Design review of the part shown in the three views and the two pictorial views. Dimensions are in mm from the part's minimum x, y and z. Give positions to 0.01 mm unless a question says otherwise; leave off trailing zeros. Write each loop counter-clockwise with the first axis right and the second up, starting at its lowest first coordinate (ties: lowest second). Pieces come first, ordered by that corner, then holes. Notation, with made-up numbers: M 43,21 L 67,21 A26 ccw 67,44 Z; hole C -11.75,-34.75 d4. An arc over 180 degrees is marked long. Write item = value, one per line.
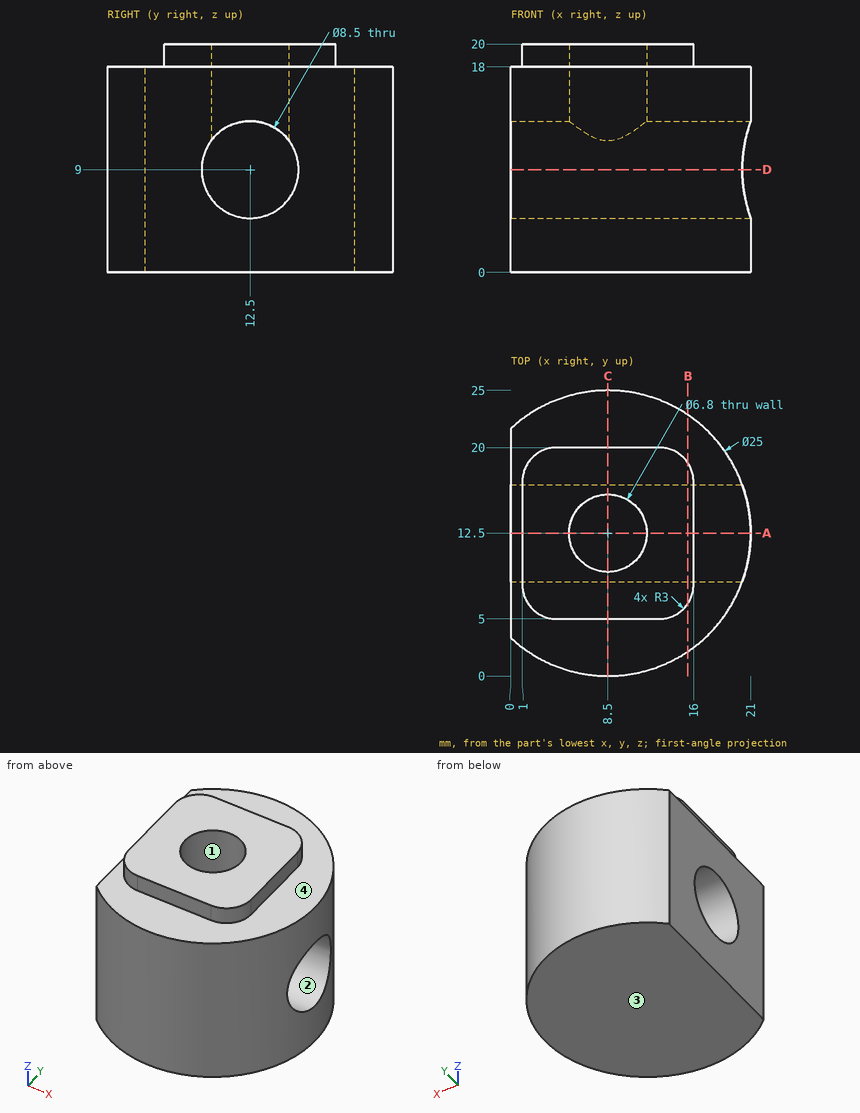
1. We need section D-D, the plane z = 9. Write out the cut boundary in (x, y).
Responses:
outline = M 0,3.33 A12.5 ccw 20.26,8.25 L 0,8.25 Z; M 0,16.75 L 20.26,16.75 A12.5 ccw 0,21.67 Z
2. Insertion check: P1, Ø2, axis at x = 7.5, y = 14, coming from the +Z side; P2, Ø10, axis at x = 2.5, z = 5, coming from the -Y side; P3, Ø6, axis at x = 15.5, z = 10.5, coming from the +Y side. Each pin has a flat end and moves straight along its axis. Give the tip position at first contact, or say it passes through.
Responses:
P1 = 5.56
P2 = 0.04
P3 = 24.34
3. The part is to be moulded in two halves that separate along Z. For the marked faces 1, 2, 3 and 4, say which applies: +Z half, -Z half, draft (parallel to the pull), parting line (faces both ways), or undercut.
Responses:
face_1 = draft
face_2 = undercut
face_3 = -Z half
face_4 = +Z half
4. For line 1 along Y through (x, z) = (8.5, 16.5); line 2 along Z through (x, y) = (4.5, 12.5); line 3 along Z through (x, y) = (1.5, 5.5), list the stretches that pass through material, from the lowest coordinate up. Write a range as from..to.
Responses:
line_1 = 0..9.1, 15.9..25
line_2 = 0..4.75, 13.25..20
line_3 = 0..18
5. We need section B-B, the plane x = 15.5. Write out the cut boundary in (y, z).
Responses:
outline = M 2.14,0 L 22.86,0 L 22.86,18 L 18.66,18 L 18.66,20 L 6.34,20 L 6.34,18 L 2.14,18 Z; hole C 12.5,9 d8.5
6. We need section A-A, the plane y = 12.5. Write out the cut boundary in (x, z).
Responses:
outline = M 0,0 L 21,0 L 21,4.75 L 0,4.75 Z; M 0,13.25 L 5.1,13.25 L 5.1,20 L 1,20 L 1,18 L 0,18 Z; M 11.9,13.25 L 21,13.25 L 21,18 L 16,18 L 16,20 L 11.9,20 Z
7. We need section C-C, the plane x = 8.5. Write out the cut boundary in (y, z), then the cut area to 3 significant figures.
Responses:
outline = M 0,0 L 25,0 L 25,18 L 20,18 L 20,20 L 15.9,20 L 15.9,11.55 A4.25 cw long 9.1,11.55 L 9.1,20 L 5,20 L 5,18 L 0,18 Z
area = 374 mm2
